```python
from build123d import *

# Parameters (mm, degrees)
SKETCH1_W               = 5.9436
SKETCH1_H               = 6.731
BOSS_EXTRUDE1_DEPTH     = 1.5875
SKETCH2_W               = 12.2936
SKETCH2_H               = 12.2936
BOSS_EXTRUDE2_DEPTH     = 3.175
SKETCH3_R               = 1.6002
CUT_EXTRUDE1_DEPTH      = 5.5593
CUT_EXTRUDE1_DEPTH_BACK = 8.7343
FILLET1_R               = 0.889
FILLET2_R               = 0.635
FILLET3_R               = 2.54
SKETCH4_W               = 1.27
SKETCH4_H               = 1.0922
CUT_EXTRUDE2_DEPTH      = 7.1468
LPATTERN1_COUNT         = 3
LPATTERN1_PITCH         = 2.1844
LPATTERN1_COL_COUNT     = 3
LPATTERN1_COL_PITCH     = 2.1844


with BuildPart() as part:
    # Sketch1 → Boss-Extrude1 (new body, symmetric)
    with BuildSketch(Plane(origin=(0, 0, 0), x_dir=(1, 0, 0), z_dir=(0, 1, 0))):
        Rectangle(SKETCH1_W, SKETCH1_H)
    extrude(amount=BOSS_EXTRUDE1_DEPTH, both=True)

    # Sketch2 → Boss-Extrude2 (add)
    with BuildSketch(Plane.XY.offset(3.3655)):
        Rectangle(SKETCH2_W, SKETCH2_H)
    extrude(amount=BOSS_EXTRUDE2_DEPTH)

    # Sketch3 → Cut-Extrude1 (cut, two sides)
    with BuildSketch(Plane(origin=(0, 1.5875, 0), x_dir=(1, 0, 0), z_dir=(0, 1, 0))) as cut_extrude1_sk:
        with Locations((0, 0.4445)):
            Circle(SKETCH3_R)
    extrude(amount=CUT_EXTRUDE1_DEPTH, mode=Mode.SUBTRACT)
    extrude(cut_extrude1_sk.sketch, amount=-CUT_EXTRUDE1_DEPTH_BACK, mode=Mode.SUBTRACT)

    # Fillet1
    fillet1_edges = [part.edges().sort_by_distance(p)[0] for p in [
        (-2.9718, 1.5875, 0),
        (2.9718, 1.5875, 0),
        (-2.9718, -1.5875, 0),
        (2.9718, -1.5875, 0),
    ]]
    fillet(fillet1_edges, radius=FILLET1_R)

    # Fillet2
    fillet2_edges = [part.edges().sort_by_distance(p)[0] for p in [
        (2.9718, 0, 3.3655),
        (0, -1.5875, 3.3655),
        (-2.9718, 0, 3.3655),
        (0, 1.5875, 3.3655),
        (2.711417928, -1.327117928, 3.3655),
        (-2.711417928, -1.327117928, 3.3655),
        (-2.711417928, 1.327117928, 3.3655),
        (2.711417928, 1.327117928, 3.3655),
    ]]
    fillet(fillet2_edges, radius=FILLET2_R)

    # Fillet3
    fillet3_edges = [part.edges().sort_by_distance(p)[0] for p in [
        (6.1468, -6.1468, 4.953),
        (6.1468, 6.1468, 4.953),
        (-6.1468, 6.1468, 4.953),
        (-6.1468, -6.1468, 4.953),
    ]]
    fillet(fillet3_edges, radius=FILLET3_R)

    # Sketch4 → Cut-Extrude2 (cut, symmetric)
    with BuildSketch(Plane(origin=(0, 0, 0), x_dir=(0, 0, -1), z_dir=(1, 0, 0))):
        with Locations((-5.9055, 0)):
            Rectangle(SKETCH4_W, SKETCH4_H)
    cut_extrude2 = extrude(amount=CUT_EXTRUDE2_DEPTH, both=True, mode=Mode.SUBTRACT)

    # LPattern1: Cut-Extrude2 ×3
    with Locations(*[(0, i * LPATTERN1_PITCH, 0) for i in range(1, LPATTERN1_COUNT)]):
        add(cut_extrude2, mode=Mode.SUBTRACT)

    # LPattern1 col: Cut-Extrude2 ×3
    with Locations(*[(0, -i * LPATTERN1_COL_PITCH, 0) for i in range(1, LPATTERN1_COL_COUNT)]):
        add(cut_extrude2, mode=Mode.SUBTRACT)


solid = part.part
```
Can you work these out from the model? Positions are in its coordinate system, mm. A direction names the side the tool comes from. Coordinates: 2 decimals unless noted, no trailing zeros. Write each loop counter-clockwise with the first axis right and the second up, starting at its lowest first coordinate (ties: lowest second). Pieces come first, ordered by that corner, then holes. Notation, with made-up numbers: M -24.75,21 L 18.25,21 A19 cw 18.25,25 Z; hole C 36,74.5 d5. An arc over 180 degrees is marked long. Write item = value, one per line. Start each with the question number.
Q1. If we section it at B-B, the plane z = 0.25: Write out the boundary of the cut face in (x, y), then the cut area to 3 significant figures.
Q2. Thinking about a two-plate mould opening in Y: for faces 1 (the face through (2.72, 1.32, -0.36)), 2 (the face through (0, 2.73, 6)), 3 (the face through (0, -3.823, 6)), 4 (the face through (6.147, 0, 5)), which applies, released by +Y, released by -Y, zero draft, split by the parting line, or undercut?
Q3. On a 3-axis mill with a long thin cutter (end or side, diameter ignored), from which of +Z, -Z, +X, -X, +Y, -Y can I reach the whole of each face in a straight line? I mean faces 5 (the face through (0, 1.638, 6)), 6 (the face through (-1, 1.588, 1)), 7 (the face through (-2.704, 1.334, -0.36)), 8 (the face through (-1, -1.588, 1)). Say none if no direction works.
Q4. If we section it at D-D, the plane z = 2.25: Write out the boundary of the cut face in (x, y), then the cut area to 3 significant figures.
Q5. If we section it at C-C, the plane y = 0.25: Write out the boundary of the cut face in (x, z) (1 decimal), then the cut area to 3 significant figures.
Q6. If I drill on L1, parallel to Z at x = 0, y = -0.25; L2, parallel to Z at x = 0, y = -0.9; L3, parallel to Y at x = 1.25, z = 1, over which ranges is the centre line in solid material (lowest first)? Write a range as [from, to].
Q7. I'm going to push flat-ended pins straight in: pin 1 (0.5 mm diameter, centred on x = 0.5, y = 0, fed in from +Z); pin 2 (3.5 mm diameter, centred on x = 0, z = -0.44, fed in from +Y); pin 3 (5 mm diameter, centred on x = 3.5, y = -5, fed in from -Z). Where does each tip first touch, or does it pass through?
Check sheet entries:
q1.outline = M -2.97,-0.7 A0.89 ccw -2.08,-1.59 L -1.44,-1.59 L -1.44,1.59 L -2.08,1.59 A0.89 ccw -2.97,0.7 Z; M 1.44,-1.59 L 2.08,-1.59 A0.89 ccw 2.97,-0.7 L 2.97,0.7 A0.89 ccw 2.08,1.59 L 1.44,1.59 Z
q1.area = 9.04 mm²
q2.face_1 = released by +Y
q2.face_2 = undercut
q2.face_3 = undercut
q2.face_4 = zero draft
q3.face_5 = +Z, +X, -X
q3.face_6 = -Z, +X, -X, +Y
q3.face_7 = -Z, -X, +Y
q3.face_8 = -Z, +X, -X, -Y
q4.outline = M -2.97,-0.7 A0.89 ccw -2.08,-1.59 L 2.08,-1.59 A0.89 ccw 2.97,-0.7 L 2.97,0.7 A0.89 ccw 2.08,1.59 L -2.08,1.59 A0.89 ccw -2.97,0.7 Z
q4.area = 18.2 mm²
q5.outline = M -6.1,3.4 L -3.6,3.4 A0.6 cw -3,2.7 L -3,-3.4 L 3,-3.4 L 3,2.7 A0.6 cw 3.6,3.4 L 6.1,3.4 L 6.1,5.3 L -6.1,5.3 Z; hole C 0,-0.4 d3.2
q5.area = 55.6 mm²
q6.L1 = [-3.37, -2.04], [1.16, 5.27]
q6.L2 = [-3.37, -2.04], [1.16, 6.54]
q6.L3 = [-1.59, 1.59]
q7.pin_1 = 5.27
q7.pin_2 = 1.59
q7.pin_3 = 3.37
